Autodesk Inventor part; units mm, degrees
ref_plane "YZ Plane" through (0, 0, 0) normal (1, 0, 0) x (0, 1, 0)
ref_plane "XZ Plane" through (0, 0, 0) normal (0, 1, 0) x (-1, 0, 0)
ref_plane "XY Plane" through (0, 0, 0) normal (0, 0, 1) x (1, 0, 0)
sketch "Sketch1" plane through (0, 0, 0) normal (0, 1, 0) x (-1, 0, 0)
  line L0 (258, 1360) -> (258, 0)
  line L1 (258, 0) -> (264, 0)
  line L2 (0, 0) -> (0, 109.131)
  line L3 (258, 1360) -> (264, 1360)
  line L4 (264, 0) -> (264, 1360)
  line L5 (263, 0) -> (259, 0)
  point P0 (261, 0)
  dimension "d3" = 6
  dimension "d5" = 1360
  dimension "d12" = 528
revolve "Revolution1" add sketch "Sketch1" angle 359.9 about axis through (0, 0, 0) along (0, 0, 1)
sketch "Sketch2" plane through (0, 0, 0) normal (0, 1, 0) x (-1, 0, 0)
  circle A0 centre (0, -706) radius 706
  point P0 (0, 0)
  dimension "d9" = 1412
extrude "Extrusion1" [suppressed]
equation "\"BendRadius\" = Thickness"
equation "\"BendReliefWidth\" = Thickness"
equation "\"BendReliefDepth\" = 0.5 * Thickness"
equation "\"CornerReliefSize\" = 4 * Thickness"
equation "\"MinimumRemnant\" = 2 * Thickness"
equation "\"TransitionRadius\" = BendRadius"
equation "\"JacobiRadiusSize\" = BendRadius"
equation "\"GapSize\" = Thickness"
properties part number "TZS 0991 accses hatch shell" material "Steel"
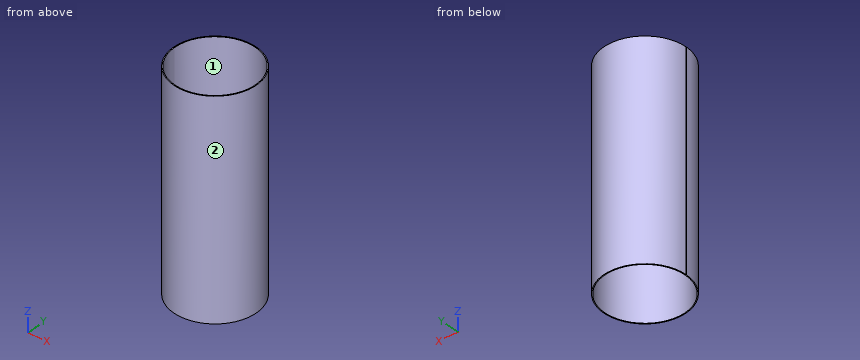
Input: part model. Units: mm. Frame: model coordinates. Face numbers are marked on the shaded views. Give positions to 0.01 mm unless a question says otherwise; leave off trailing zeros. Order: outer loops, then holes, each group sorted by start corner. A loop starts at its lowest first (then second) coordinate and runs counter-clockwise, first axis right, second up.
Q1. Section C-C on z = 118. Output: boundary loops of the cut face in (x, y).
Checked values:
outline: (-264, 0) arc R264 ccw (long way) to (-264, 0.46) - (-258, 0.45) arc R258 cw (long way) to (-258, 0) - close
Q2. Draft query along Y for the marked faces 1 and 2. Return one class per face: +Y half, -Y half, draft (parallel to the pull), parting line (faces both ways), or undercut.
Checked values:
face 1: undercut
face 2: parting line
Q3. Section B-B on y = -87. Output: boundary loops of the cut face in (x, z).
Checked values:
outline: (-249.25, 0) - (-242.89, 0) - (-242.89, 1360) - (-249.25, 1360) - close; (242.89, 0) - (249.25, 0) - (249.25, 1360) - (242.89, 1360) - close
Q4. Section A-A on x = 0. Output: boundary loops of the cut face in (y, z), and give its area (3 significant figures).
Checked values:
outline: (-264, 0) - (-258, 0) - (-258, 1360) - (-264, 1360) - close; (258, 0) - (264, 0) - (264, 1360) - (258, 1360) - close
area: 16,300 mm2
Q5. Ray query, probe 1 along Y at (x, z) = (0, 986); probe 2 along X at (y, z) = (-188, 896). Return the intervals inside material, ascending.
Checked values:
probe 1: y = -264 to -258, 258 to 264
probe 2: x = -185.34 to -176.69, 176.69 to 185.34
Q6. Contact query for flat-ended pins moving along their axis: pin 1 Ø1 at (x, z) = (144.5, 981) entering from +Y; pin 2 Ø4 at (x, z) = (-69, 379.5) entering from +Y; pin 3 Ø5 at (x, z) = (-72.5, 1123) entering from -Y. Output: stop coordinate, or through.
Checked values:
pin 1: stops at y = 221.27
pin 2: stops at y = 255.36
pin 3: stops at y = -254.55
